Design review of the part built by this model. Coordinates are the model's own, in mm. A direction names the side the tool comes from. Give positions to 0.01 mm unless a question says otherwise; leave off trailing zeros. Order: outer loops, then holes, each group sorted by start corner. A loop starts at its lowest first (then second) coordinate and runs counter-clockwise, first axis right, second up. Notation, with made-up numbers: M 35.5,55.5 L 56.5,55.5 A18 ccw 56.5,86.5 Z; hole C -27.75,31 d6. An arc over 180 degrees is marked long. Answer as a JSON object with one key per item and string values.
from build123d import *

# Parameters (mm, degrees)
BOSS_EXTRUDE1_DEPTH          = 4.7625
FILLET5_R                    = 4.7625
F_97_0_0059_DIAMETER_HOLE1_D = 5.499999922
CUT_EXTRUDE1_DEPTH           = 2.38125
F_8_CLEARANCE_HOLE1_D        = 4.4958


with BuildPart() as part:
    # Sketch1 → Boss-Extrude1 (new body)
    with BuildSketch(Plane(origin=(0, 0, 0), x_dir=(1, 0, 0), z_dir=(0, 1, 0))):
        Polygon((-6.35, 193.821953186), (126.116733726, -6.35), (-6.35, -6.35), align=None)
        with BuildLine():
            Line((51.297931724, 83.696727765), (102.483266274, 6.35))
            Line((102.483266274, 6.35), (6.35, 6.35))
            Line((6.35, 6.35), (6.35, 151.618046814))
            Line((6.35, 151.618046814), (39.158490531, 102.040772235))
            ThreePointArc((39.158490531, 102.040772235), (40.201209552, 98.92354296), (39.545616076, 95.702583707))
            ThreePointArc((39.545616076, 95.702583707), (39.932741621, 89.36439518), (45.615336672, 86.530561472))
            ThreePointArc((45.615336672, 86.530561472), (48.836295925, 85.874967996), (51.297931724, 83.696727765))
        make_face(mode=Mode.SUBTRACT)
    extrude(amount=BOSS_EXTRUDE1_DEPTH)

    # Fillet5
    fillet5_edges = [part.edges().sort_by_distance(p)[0] for p in [
        (6.35, 2.38125, -151.618046814),
        (6.35, 2.38125, -6.35),
        (102.483266274, 2.38125, -6.35),
        (-6.35, 2.38125, -193.821953186),
        (126.116733726, 2.38125, 6.35),
        (-6.35, 2.38125, 6.35),
    ]]
    fillet(fillet5_edges, radius=FILLET5_R)

    # #97 (0.0059) Diameter Hole1 (through all)
    with Locations(Plane(origin=(0, 4.7625, 0), x_dir=(1, 0, 0), z_dir=(0, 1, 0))):
        with Locations((0, 172.72), (0, 0), (113.792, 0)):
            Hole(F_97_0_0059_DIAMETER_HOLE1_D / 2)

    # Sketch5 → Cut-Extrude1 (cut)
    with BuildSketch(Plane(origin=(0, 4.7625, 0), x_dir=(1, 0, 0), z_dir=(0, 1, 0))):
        with BuildLine():
            Line((110.252008963, 8.993563641), (6.506878053, 165.763983683))
            ThreePointArc((6.506878053, 165.763983683), (4.750358466, 167.059159309), (2.5727622, 166.914537515))
            ThreePointArc((2.5727622, 166.914537515), (1.829790785, 166.639344963), (1.058333333, 166.458815563))
            ThreePointArc((1.058333333, 166.458815563), (-0.837446305, 165.377677032), (-1.5875, 163.328223344))
            Line((-1.5875, 163.328223344), (-1.5875, 9.391776656))
            ThreePointArc((-1.5875, 9.391776656), (-0.837446305, 7.342322968), (1.058333333, 6.261184437))
            ThreePointArc((1.058333333, 6.261184437), (4.490128061, 4.490128061), (6.261184437, 1.058333333))
            ThreePointArc((6.261184437, 1.058333333), (7.342322968, -0.837446305), (9.391776656, -1.5875))
            Line((9.391776656, -1.5875), (104.400223344, -1.5875))
            ThreePointArc((104.400223344, -1.5875), (106.449677032, -0.837446305), (107.530815563, 1.058333333))
            ThreePointArc((107.530815563, 1.058333333), (108.267435402, 3.130764444), (109.666849473, 4.827590821))
            ThreePointArc((109.666849473, 4.827590821), (110.748409623, 6.799755727), (110.252008963, 8.993563641))
        make_face()
    extrude(amount=-CUT_EXTRUDE1_DEPTH, mode=Mode.SUBTRACT)

    # #8 Clearance Hole1 (through all)
    with Locations(Plane(origin=(0, 2.38125, 0), x_dir=(1, 0, 0), z_dir=(0, 1, 0))):
        with Locations((2.9845, 92.075), (43.1165, 92.075)):
            Hole(F_8_CLEARANCE_HOLE1_D / 2)


solid = part.part
(1) Draft analysis for pull direction Z (two halves, no side actions). For faces 4 (the flat face through (53, 0, -82)), 5 (the flat face through (60.973, 2.348, -92.089)), 6 (the cylindrical face through (-1.27, 2.35, 2.44)), 7 (the cylindrical face through (-4.99, 2.41, 4.92)), state which applies: +Z half, -Z half, draft (parallel to the pull), parting line (faces both ways), or undercut.
Checked values:
{"face 4": "draft", "face 5": "-Z half", "face 6": "undercut", "face 7": "+Z half"}
(2) Tool access review of faces 1 (the flat face through (63, 4.762, -82)), 2 (the flat face through (74.12, 1.17, -49.21)), 3 (the flat face through (42, 2.381, -89)): name each direction out of +Z, -Z, +X, -X, +Y, -Y from which nothing blocks a thin tool from reaching the whole face with its end or side.
Checked values:
{"face 1": "+Z, -Z, +X, -X, +Y", "face 2": "+Y, -Y", "face 3": "+Y"}
(3) We need section D-D (z = -142.5). Write out the cut boundary in (x, y).
Checked values:
{"outline": "M -6.35,0 L 27.61,0 L 27.61,4.76 L 21.9,4.76 L 21.9,2.38 L -1.59,2.38 L -1.59,4.76 L -6.35,4.76 Z"}
(4) Insertion check: pin 1 (1 mm diameter, centred on y = 4, z = -133, fed in from +X); pin 2 (1.2 mm diameter, centred on y = 1.5, z = -102.5, fed in from +X); pin 3 (0.7 mm diameter, centred on x = 34, y = 3, fed in from -Z); pin 4 (7 mm diameter, centred on x = 0, z = 0, fed in from -Y). Each pin has a flat end and moves straight along its axis. Give the tip position at first contact, or say it passes through.
Checked values:
{"pin 1": "stops at x = 34.23", "pin 2": "stops at x = 54.48", "pin 3": "stops at z = -133.38", "pin 4": "stops at y = 0"}
(5) We need section A-A (x = 28.5). Write out the cut boundary in (y, z).
Checked values:
{"outline": "M 0,-141.16 L 4.76,-141.16 L 4.76,-132.53 L 2.38,-132.53 L 2.38,-118.15 L 0,-118.15 Z; M 0,-6.35 L 2.38,-6.35 L 2.38,1.59 L 4.76,1.59 L 4.76,6.35 L 0,6.35 Z"}
(6) To check wall thickness, follow L1, parallel to Z at x = 0.5, y = 4.15; L2, parallel to X at y = 1.65, z = -91; L3, parallel to Z at x = 0, y = 1.65. State the ranges of each line that lie inside material, in increasing order. Write a range as from..to.
Checked values:
{"L1": "z = -182.28..-175.42, -170.02..-166.31, -6.41..-2.7, 2.7..6.35", "L2": "x = -6.35..1.01, 4.96..6.35, 39.16..41.14, 45.09..61.69", "L3": "z = -182.49..-175.47, -169.97..-2.75, 2.75..6.35"}
(7) We need section C-C (y = 1.45). Count the separate pieces of the cut face and the enclosed holes in it, plus the area to 3 significant figures.
Checked values:
{"separate pieces": "1", "enclosed holes": "6", "area": "6,240 mm^2"}
(8) We need section B-B (z = -172.72). Write out the cut boundary in (x, y).
Checked values:
{"outline": "M -6.35,0 L -2.75,0 L -2.75,4.76 L -6.35,4.76 Z; M 2.75,0 L 7.61,0 L 7.61,4.76 L 2.75,4.76 Z"}
